```python
from build123d import *

# Parameters (mm, degrees)
SKETCH_1_W           = 21
SKETCH_1_H           = 10
EXTRUDE_1_DEPTH      = 1
SKETCH_2_R           = 1.2
EXTRUDE_2_DEPTH      = 2
SKETCH_3_R           = 0.85
CUT_EXTRUDE_2_DEPTH  = 3
EXTRUDE_3_DEPTH      = 0.5
EXTRUDE_3_DEPTH_BACK = 2
SKETCH_5_R           = 0.9
SKETCH_7_R           = 2
CUT_EXTRUDE_4_DEPTH  = 1
SKETCH_8_R           = 0.5
CUT_EXTRUDE_5_DEPTH  = 1
SKETCH_9_R           = 0.5
CUT_EXTRUDE_6_DEPTH  = 2
SKETCH_10_R          = 1
EXTRUDE_4_DEPTH      = 1
CUT_EXTRUDE_START    = -1
SKETCH_11_R          = 0.5
CUT_EXTRUDE_7_DEPTH  = 1


with BuildPart() as part:
    # 草图1 → 凸台-拉伸1 (new body)
    with BuildSketch(Plane(origin=(0, 0, 0), x_dir=(1, 0, 0), z_dir=(0, 1, 0))):
        Rectangle(SKETCH_1_W, SKETCH_1_H)
    extrude(amount=EXTRUDE_1_DEPTH)

    # 草图2 → 凸台-拉伸2 (add)
    with BuildSketch(Plane(origin=(0, 1, 0), x_dir=(1, 0, 0), z_dir=(0, 1, 0))):
        with Locations(Location((5.2, -0.2, 0), (0, 0, 270))):
            Circle(SKETCH_2_R)
    extrude(amount=EXTRUDE_2_DEPTH)

    # 草图3 → 切除-拉伸2 (cut)
    with BuildSketch(Plane(origin=(0, 3, 0), x_dir=(1, 0, 0), z_dir=(0, 1, 0))):
        with Locations(Location((5.2, -0.2, 0), (0, 0, 270))):
            Circle(SKETCH_3_R)
    extrude(amount=-CUT_EXTRUDE_2_DEPTH, mode=Mode.SUBTRACT)

    # 草图5 → 凸台-拉伸3 (add, two sides: drawn at the far end of the back side and taken through both)
    with BuildSketch(Plane(origin=(0, 1, 0), x_dir=(1, 0, 0), z_dir=(0, 1, 0)).offset(-EXTRUDE_3_DEPTH_BACK)):
        with Locations(Location((-1.05, -0.2, 0), (0, 0, 270))):
            Circle(SKETCH_5_R)
    extrude(amount=EXTRUDE_3_DEPTH + EXTRUDE_3_DEPTH_BACK)

    # 草图7 → 切除-拉伸4 (cut)
    with BuildSketch(Plane(origin=(0, 1, 0), x_dir=(1, 0, 0), z_dir=(0, 1, 0))):
        with Locations(Location((-6.75, -0.2, 0), (0, 0, 270))):
            Circle(SKETCH_7_R)
    extrude(amount=-CUT_EXTRUDE_4_DEPTH, mode=Mode.SUBTRACT)

    # 草图8 → 切除-拉伸5 (cut)
    with BuildSketch(Plane(origin=(0, 1, 0), x_dir=(1, 0, 0), z_dir=(0, 1, 0))):
        with Locations(Location((9, 3.5, 0), (0, 0, 270))):
            Circle(SKETCH_8_R)
        with Locations(Location((1, 3.5, 0), (0, 0, 270))):
            Circle(SKETCH_8_R)
        with Locations(Location((9, -3.5, 0), (0, 0, 270))):
            Circle(SKETCH_8_R)
    extrude(amount=-CUT_EXTRUDE_5_DEPTH, mode=Mode.SUBTRACT)

    # 草图9 → 切除-拉伸6 (cut)
    with BuildSketch(Plane(origin=(0, 1.5, 0), x_dir=(1, 0, 0), z_dir=(0, 1, 0))):
        with Locations(Location((-1.05, -0.2, 0), (0, 0, 270))):
            Circle(SKETCH_9_R)
    extrude(amount=-CUT_EXTRUDE_6_DEPTH, mode=Mode.SUBTRACT)

    # 草图10 → 凸台-拉伸4 (add)
    with BuildSketch(Plane.XZ):
        with Locations(Location((9, 3.5, 0), (0, 0, 90))):
            Circle(SKETCH_10_R)
        with Locations(Location((9, -3.5, 0), (0, 0, 90))):
            Circle(SKETCH_10_R)
        with Locations(Location((1, -3.5, 0), (0, 0, 90))):
            Circle(SKETCH_10_R)
    extrude(amount=EXTRUDE_4_DEPTH)

    # 草图11 → 切除-拉伸7 (cut)
    with BuildSketch(Plane.XZ.offset(1).offset(CUT_EXTRUDE_START)):
        with Locations(Location((9, 3.5, 0), (0, 0, 90))):
            Circle(SKETCH_11_R)
        with Locations(Location((9, -3.5, 0), (0, 0, 90))):
            Circle(SKETCH_11_R)
        with Locations(Location((1, -3.5, 0), (0, 0, 90))):
            Circle(SKETCH_11_R)
    extrude(amount=CUT_EXTRUDE_7_DEPTH, mode=Mode.SUBTRACT)


solid = part.part
```
CAD build for the part. Positions are in the model's coordinates, mm. A direction names the side the tool comes from. Round coordinates to 2 decimals unless told otherwise and drop trailing zeros. Loops run counter-clockwise (first coordinate to the right, second up) from the corner with the lowest first, then second, coordinate; pieces in that order, holes last. Notation, with made-up numbers: M 30.25,-23.5 L 72.25,-23.5 A22 ccw 72.25,-15.5 Z; hole C 23.25,-24 d3. An arc over 180 degrees is marked long. Use a Markdown table: item, result. Add a question column.
(1) Pull direction Z, two halves, no side cores. Call faces 4 (the face through (-1, -1, 0)), 5 (the face through (-5.398, 0.507, -1.274)), 6 (the face through (-0.1, 0.5, -5)): +Z half, -Z half, draft (parallel to the pull), parting line (faces both ways), or undercut.
(2) Cut at D-D (x = 1). Give the cut face in (y, z), and give its area (3 significant figures).
(3) Drill centre lines: line 1 (Z direction, x = 9, y = -0.6); line 2 (X direction, y = -0.8, z = -3.5); line 3 (X direction, y = 0.65, z = 0). Where is each one in solid material? Low to high.
(4) Cut at C-C (y = 0.4). Give the cut face in (x, z).
(5) Flat gauge pins, fed straight in: pin 1 (3 mm diameter, centred on x = -4, z = -1, fed in from +Y); pin 2 (0.8 mm diameter, centred on x = -1, z = 0.5, fed in from +Y); pin 3 (1.4 mm diameter, centred on x = 5.2, z = 0.2, fed in from -Y) (3 decimals); pin 4 (1.5 mm diameter, centred on x = 4.5, y = 1.5, fed in from +Z). Where does each tip first touch, or does it go through?
(6) Cut at B-B (z = -3.5). Give the cut face in (x, y), and give its area (3 significant figures).
(7) Cut at A-A (x = 9). Give the cut face in (y, z), and give its area (3 significant figures).
(8) Which spindle directions (+Z, -Z, +X, -X, +Y, -Y) get a long thin tool onto all of the face, cutting with end or side? Do faces 1 (the face through (8.01, -0.49, 3.37)), 2 (the face through (-0.1, 0.5, 5)), 3 (the face through (6.21, 1.99, 0.85)). Say none if no direction does.
Geometry says:
| question | item | result |
|---|---|---|
| 1 | face 4 | draft |
| 1 | face 5 | undercut |
| 1 | face 6 | -Z half |
| 2 | outline | M -1,-4.5 L 0,-4.5 L 0,-5 L 1,-5 L 1,-4 L -1,-4 Z; M -1,-3 L 1,-3 L 1,5 L 0,5 L 0,-2.5 L -1,-2.5 Z |
| 2 | area | 10.0 mm² |
| 3 | line 1 | z = -4.5 to -4, -3 to -2.5, 2.5 to 3, 4 to 4.5 |
| 3 | line 2 | x = 0 to 0.5, 1.5 to 2, 8 to 8.5, 9.5 to 10 |
| 3 | line 3 | x = -10.5 to -8.74, -4.76 to -1.51, -0.59 to 4.37, 6.03 to 10.5 |
| 4 | outline | M -10.5,-5 L 10.5,-5 L 10.5,5 L -10.5,5 Z; hole C -6.75,0.2 d4; hole C -1.05,0.2 d1; hole C 1,-3.5 d1; hole C 5.2,0.2 d1.7; hole C 9,-3.5 d1; hole C 9,3.5 d1 |
| 5 | pin 1 | stops at y = 1 |
| 5 | pin 2 | stops at y = 1.5 |
| 5 | pin 3 | passes through |
| 5 | pin 4 | stops at z = 5 |
| 6 | outline | M -10.5,0 L 0,0 L 0,-1 L 0.5,-1 L 0.5,1 L -10.5,1 Z; M 1.5,-1 L 2,-1 L 2,0 L 8,0 L 8,-1 L 8.5,-1 L 8.5,1 L 1.5,1 Z; M 9.5,-1 L 10,-1 L 10,0 L 10.5,0 L 10.5,1 L 9.5,1 Z |
| 6 | area | 21.0 mm² |
| 7 | outline | M -1,-4.5 L 0,-4.5 L 0,-5 L 1,-5 L 1,-4 L -1,-4 Z; M -1,-3 L 1,-3 L 1,3 L -1,3 L -1,2.5 L 0,2.5 L 0,-2.5 L -1,-2.5 Z; M -1,4 L 1,4 L 1,5 L 0,5 L 0,4.5 L -1,4.5 Z |
| 7 | area | 10.0 mm² |
| 8 | face 1 | -Y |
| 8 | face 2 | +Z, +X, -X, +Y, -Y |
| 8 | face 3 | +Y |
